Model file for the job. Use its own axes, mm. A direction names the side the tool comes from. Coordinates: 2 decimals unless noted, no trailing zeros. Order: outer loops, then holes, each group sorted by start corner. A loop starts at its lowest first (then second) coordinate and runs counter-clockwise, first axis right, second up. Notation, with made-up numbers: M 73,6 L 89,6 A10 ccw 89,16 Z; hole C 13,-10 d3. An arc over 180 degrees is marked long. Return JSON: item names as keys, results as strings.
```python
from build123d import *

# Parameters (mm, degrees)
ESQUISSE1_W             = 30
ESQUISSE1_H             = 70
ESQUISSE1_R             = 1.5
ESQUISSE1_W_2           = 3
ESQUISSE1_H_2           = 5
BOSS_EXTRU_1_DEPTH      = 5
ESQUISSE2_W             = 8.5
ESQUISSE2_H             = 3
ENL_V_MAT_EXTRU_1_DEPTH = 5
ESQUISSE3_W             = 30
ESQUISSE3_H             = 5
BOSS_EXTRU_2_DEPTH      = 5
ESQUISSE4_R             = 1.05
ENL_V_MAT_EXTRU_2_DEPTH = 10


with BuildPart() as part:
    # Esquisse1 → Boss.-Extru.1 (new body)
    with BuildSketch(Plane.XY):
        with Locations((15, 35)):
            Rectangle(ESQUISSE1_W, ESQUISSE1_H)
        with Locations((15, 5)):
            Circle(ESQUISSE1_R, mode=Mode.SUBTRACT)
        with Locations((15, 13.5)):
            Circle(ESQUISSE1_R, mode=Mode.SUBTRACT)
        with Locations((15, 22)):
            Circle(ESQUISSE1_R, mode=Mode.SUBTRACT)
        with Locations((12.5, 35.4)):
            Rectangle(ESQUISSE1_W_2, ESQUISSE1_H_2, mode=Mode.SUBTRACT)
        with Locations((7.5, 35.4)):
            Rectangle(ESQUISSE1_W_2, ESQUISSE1_H_2, mode=Mode.SUBTRACT)
        with Locations((17.5, 35.4)):
            Rectangle(ESQUISSE1_W_2, ESQUISSE1_H_2, mode=Mode.SUBTRACT)
        with Locations((22.5, 35.4)):
            Rectangle(ESQUISSE1_W_2, ESQUISSE1_H_2, mode=Mode.SUBTRACT)
        with Locations((22.5, 62.6)):
            Rectangle(ESQUISSE1_W_2, ESQUISSE1_H_2, mode=Mode.SUBTRACT)
        with Locations((17.5, 62.6)):
            Rectangle(ESQUISSE1_W_2, ESQUISSE1_H_2, mode=Mode.SUBTRACT)
        with Locations((12.5, 62.6)):
            Rectangle(ESQUISSE1_W_2, ESQUISSE1_H_2, mode=Mode.SUBTRACT)
        with Locations((7.5, 62.6)):
            Rectangle(ESQUISSE1_W_2, ESQUISSE1_H_2, mode=Mode.SUBTRACT)
    extrude(amount=BOSS_EXTRU_1_DEPTH)

    # Esquisse2 → Enlèv. mat.-Extru.1 (cut)
    with BuildSketch(Plane.XY.offset(5)):
        with Locations((15, 39.4)):
            Rectangle(ESQUISSE2_W, ESQUISSE2_H)
    extrude(amount=-ENL_V_MAT_EXTRU_1_DEPTH, mode=Mode.SUBTRACT)

    # Esquisse3 → Boss.-Extru.2 (add)
    with BuildSketch(Plane(origin=(0, 70, 0), x_dir=(1, 0, 0), z_dir=(0, 1, 0))):
        with Locations((15, -2.5)):
            Rectangle(ESQUISSE3_W, ESQUISSE3_H)
    extrude(amount=BOSS_EXTRU_2_DEPTH)

    # Esquisse4 → Enlèv. mat.-Extru.2 (cut)
    with BuildSketch(Plane.XY.offset(5)):
        with Locations((15, 71.1)):
            Circle(ESQUISSE4_R)
    extrude(amount=-ENL_V_MAT_EXTRU_2_DEPTH, mode=Mode.SUBTRACT)


solid = part.part
```
Item 1: Drop flat-ended pins along their axis: pin 1 Ø1.3 at (x, y) = (15, 71.1) entering from +Z; pin 2 Ø0.9 at (x, z) = (17, 3.5) entering from -Y. Give the stop position or say it passes through.
Check result:
{"pin 1": "passes through", "pin 2": "stops at y = 0"}
Item 2: Saw through at C-C (z = 1.95). Count the separate pieces of the cut face and the enclosed holes in it, and give its area (3 significant figures).
Check result:
{"separate pieces": "1", "enclosed holes": "11", "area": "2,080 mm2"}
Item 3: Saw through at A-A (y = 5). Write the cut outline in (x, z), and give its area (3 significant figures).
Check result:
{"outline": "M 0,0 L 13.5,0 L 13.5,5 L 0,5 Z; M 16.5,0 L 30,0 L 30,5 L 16.5,5 Z", "area": "135 mm2"}
Item 4: Saw through at B-B (y = 62). Write the cut outline in (x, z).
Check result:
{"outline": "M 0,0 L 6,0 L 6,5 L 0,5 Z; M 9,0 L 11,0 L 11,5 L 9,5 Z; M 14,0 L 16,0 L 16,5 L 14,5 Z; M 19,0 L 21,0 L 21,5 L 19,5 Z; M 24,0 L 30,0 L 30,5 L 24,5 Z"}
Item 5: Wall check: line 1 (Y direction, x = 11.75, z = 4.7); line 2 (Y direction, x = 15, z = 2.95); line 3 (Y direction, x = 23.25, z = 3.1). Give the ranges that are in metal, low to high.
Check result:
{"line 1": "y = 0 to 32.9, 40.9 to 60.1, 65.1 to 75", "line 2": "y = 0 to 3.5, 6.5 to 12, 15 to 20.5, 23.5 to 37.9, 40.9 to 70.05, 72.15 to 75", "line 3": "y = 0 to 32.9, 37.9 to 60.1, 65.1 to 75"}
Item 6: 3-axis set-ups, long thin cutter, end or side, ignore diameter. For faces 1 (the flat face through (12, 60.1, 2)), 2 (the flat face through (15, 75, 2)): which of +Z, -Z, +X, -X, +Y, -Y reach the whole face in a straight line?
Check result:
{"face 1": "+Z, -Z", "face 2": "+Z, -Z, +X, -X, +Y"}
Item 7: Pull direction X, two halves, no side cores. Call faces 3 (the flat face through (15, 37, 0)), 4 (the flat face through (17, 32.9, 2)): +X half, -X half, draft (parallel to the pull), parting line (faces both ways), or undercut.
Check result:
{"face 3": "draft", "face 4": "undercut"}
Item 8: Saw through at D-D (y = 71.1). Write the cut outline in (x, z).
Check result:
{"outline": "M 0,0 L 13.95,0 L 13.95,5 L 0,5 Z; M 16.05,0 L 30,0 L 30,5 L 16.05,5 Z"}
